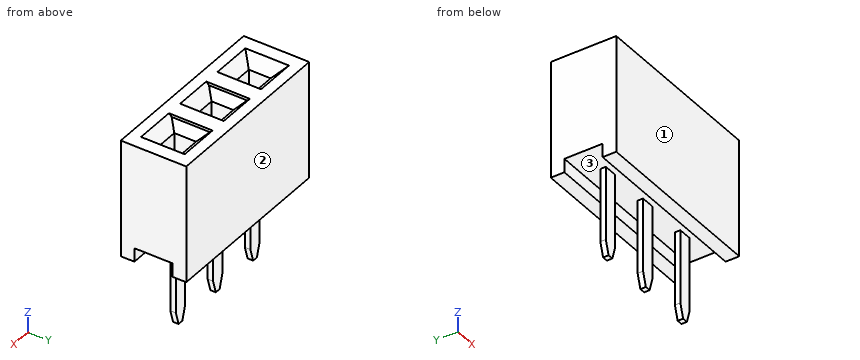
from build123d import *

# Parameters (mm, degrees)
SKETCH1_W           = 2.4
SKETCH1_H           = 4.3
BOSS_EXTRUDE1_DEPTH = 1.3
SKETCH_1_W          = 0.5
SKETCH_1_H          = 1.4
CUT_EXTRUDE_1_DEPTH = 6.166236541
SKETCH2_W           = 0.8
SKETCH2_H           = 0.8
CUT_EXTRUDE1_DEPTH  = 3.1
CHAMFER_1_SIZE      = 0.4
BOSS_EXTRUDE2_DEPTH = 0.1
LPATTERN1_COUNT     = 3
LPATTERN1_PITCH     = 2


with BuildPart() as part:
    # Sketch1 → Boss-Extrude1 (new, symmetric)
    with BuildSketch(Plane(origin=(0, 0, 0), x_dir=(0, -1, 0), z_dir=(1, 0, 0))):
        with Locations((0, -2.15)):
            Rectangle(SKETCH1_W, SKETCH1_H)
    extrude(amount=BOSS_EXTRUDE1_DEPTH, both=True)

    # Эскиз1 → Вырез-Вытянуть1 (cut, through all)
    with BuildSketch(Plane(origin=(1.3, 0, 0), x_dir=(0, 0, -1), z_dir=(1, 0, 0))):
        with Locations((-0.25, 0)):
            Rectangle(SKETCH_1_W, SKETCH_1_H)
    extrude(amount=-CUT_EXTRUDE_1_DEPTH, mode=Mode.SUBTRACT)

    # Sketch2 → Cut-Extrude1 (cut)
    with BuildSketch(Plane(origin=(0, 0, 4.3), x_dir=(-1, 0, 0), z_dir=(0, 0, 1))):
        Rectangle(SKETCH2_W, SKETCH2_H)
    extrude(amount=-CUT_EXTRUDE1_DEPTH, mode=Mode.SUBTRACT)

    # Фаска1
    chamfer_1_edges = [part.edges().sort_by_distance(p)[0] for p in [
        (-0.4, 0, 4.3),
        (0, -0.4, 4.3),
        (0.4, 0, 4.3),
        (0, 0.4, 4.3),
    ]]
    chamfer(chamfer_1_edges, length=CHAMFER_1_SIZE)

    # Sketch3 → Boss-Extrude2 (add, symmetric)
    with BuildSketch(Plane(origin=(0, 0, 0), x_dir=(1, 0, 0), z_dir=(0, 1, 0))):
        Polygon((-0.25, 0), (-0.25, 2.2), (-0.1, 2.7), (0.1, 2.7), (0.25, 2.2), (0.25, 0), (0.25, -0.5), (-0.25, -0.5), align=None)
        Polygon((0.4, -1.2), (-0.4, -1.2), (-0.4, -3.1), (-0.3, -3.1), (-0.3, -1.3), (0.3, -1.3), (0.3, -3.1), (0.4, -3.1), align=None)
    extrude(amount=BOSS_EXTRUDE2_DEPTH, both=True)


with BuildPart() as lpattern1_1:
    # LPattern1: pattern copy
    add(part.part.moved(Location(Vector(1, 0, 0) * (1 * LPATTERN1_PITCH))))


with BuildPart() as lpattern1_2:
    # LPattern1: pattern copy
    add(part.part.moved(Location(Vector(1, 0, 0) * (2 * LPATTERN1_PITCH))))


with BuildPart() as lpattern1_1_1:
    add(lpattern1_1.part)

    # Combine 1: union part, LPattern1_2
    add(part.part)
    add(lpattern1_2.part)


solid = lpattern1_1_1.part
Input: part model. Units: mm. Frame: model coordinates. Face numbers are marked on the shaded views. Give positions to 0.01 mm unless a question says otherwise; leave off trailing zeros. Order: outer loops, then holes, each group sorted by start corner. A loop starts at its lowest first (then second) coordinate and runs counter-clockwise, first axis right, second up.
Q1. Section A-A on z = -1.25. Output: boundary loops of the cut face in (x, y).
Checked values:
outline: (-0.25, -0.1) - (0.25, -0.1) - (0.25, 0.1) - (-0.25, 0.1) - close; (1.75, -0.1) - (2.25, -0.1) - (2.25, 0.1) - (1.75, 0.1) - close; (3.75, -0.1) - (4.25, -0.1) - (4.25, 0.1) - (3.75, 0.1) - close
Q2. Section C-C on y = 0.55. Output: boundary loops of the cut face in (x, z), and give its area (3 significant figures).
Checked values:
outline: (-1.3, 0.5) - (5.3, 0.5) - (5.3, 4.3) - (4.8, 4.3) - (4.55, 4.05) - (3.45, 4.05) - (3.3, 4.2) - (3.3, 4.3) - (2.7, 4.3) - (2.7, 4.2) - (2.55, 4.05) - (1.45, 4.05) - (1.3, 4.2) - (1.3, 4.3) - (0.7, 4.3) - (0.7, 4.2) - (0.55, 4.05) - (-0.55, 4.05) - (-0.8, 4.3) - (-1.3, 4.3) - close
area: 24.1 mm2
Q3. Section B-B on x = 4.5. Output: boundary loops of the cut face in (y, z), and give its area (3 significant figures).
Checked values:
outline: (-1.2, 0) - (-0.7, 0) - (-0.7, 0.5) - (0.7, 0.5) - (0.7, 0) - (1.2, 0) - (1.2, 4.3) - (0.8, 4.3) - (0.5, 4) - (-0.5, 4) - (-0.8, 4.3) - (-1.2, 4.3) - close
area: 9.23 mm2
Q4. Ray query, probe 1 along X at (y, z) = (0.35, 3.5); probe 2 along Y at (x, z) = (3.75, 3.25); probe 3 along Z at (x, y) = (1, -0.85). Return the intervals inside material, ascending.
Checked values:
probe 1: x = -1.3 to -0.4, 0.4 to 1.6, 2.4 to 3.6, 4.4 to 5.3
probe 2: y = -1.2 to -0.4, 0.4 to 1.2
probe 3: z = 0 to 4.3
Q5. Draft query along Y for the marked faces 1, 2 and 3. Return one class per face: +Y half, -Y half, draft (parallel to the pull), parting line (faces both ways), or undercut.
Checked values:
face 1: -Y half
face 2: +Y half
face 3: undercut
Q6. Section D-D on z = 2. State how many separate pieces and enclosed holes the cut face has, and give its area (3 significant figures).
Checked values:
separate pieces: 1
enclosed holes: 3
area: 14.0 mm2
